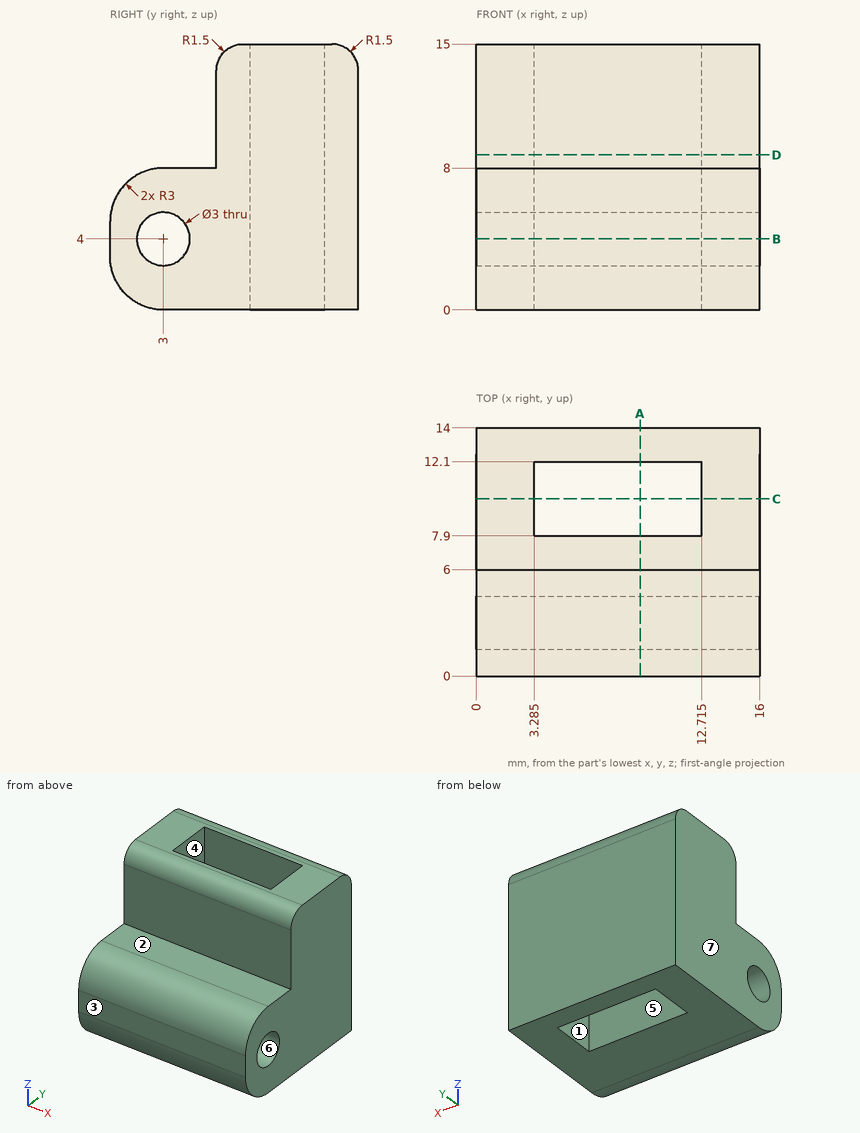
Source: three-view drawing plus pictorial views. Frame: mm from the lowest corner of the part. A direction names the side the tool comes from. Coordinates: 2 decimals unless noted, no trailing zeros. Order: outer loops, then holes, each group sorted by start corner. A loop starts at its lowest first (then second) coordinate and runs counter-clockwise, first axis right, second up. Notation, with made-up numbers: M -37.75,67.25 L 15.25,67.25 A13 ccw 15.25,81.25 Z; hole C 12.25,-34.75 d4. An arc over 180 degrees is marked long. Answer in a Markdown table with one row per item.
(1) Section query A-A, the plane x = 9.25. Output: boundary loops of the cut face in (y, z), plus the area to 3 significant figures.
Numbers:
| item | result |
|---|---|
| outline | M 0,3 A3 ccw 3,0 L 7.9,0 L 7.9,15 L 7.5,15 A1.5 ccw 6,13.5 L 6,8 L 3,8 A3 ccw 0,5 Z; M 12.1,0 L 14,0 L 14,13.5 A1.5 ccw 12.5,15 L 12.1,15 Z; hole C 3,4 d3 |
| area | 93.1 mm^2 |
(2) Section query B-B, the plane z = 4. Output: boundary loops of the cut face in (x, y) (3 decimals), plus the area to 3 significant figures.
Numbers:
| item | result |
|---|---|
| outline | M 0,0 L 16,0 L 16,1.5 L 0,1.5 Z; M 0,4.5 L 16,4.5 L 16,14 L 0,14 Z; hole M 3.285,7.9 L 12.715,7.9 L 12.715,12.1 L 3.285,12.1 Z |
| area | 136 mm^2 |
(3) Access query for the marked faces 1, 2 and 3. Directions: +Z, -Z, +X, -X, +Y, -Y. A direction counts if a zero-diameter tool reaches every point of the face in a straight line with its end or side. Return the directions, or none.
Numbers:
| item | result |
|---|---|
| face 1 | +Z, -Z |
| face 2 | +Z, +X, -X, -Y |
| face 3 | +Z, -Z, +X, -X, -Y |
(4) Section query D-D, the plane z = 8.75. Output: boundary loops of the cut face in (x, y) (3 decimals).
Numbers:
| item | result |
|---|---|
| outline | M 0,6 L 16,6 L 16,14 L 0,14 Z; hole M 3.285,7.9 L 12.715,7.9 L 12.715,12.1 L 3.285,12.1 Z |
(5) Contact query for flat-ended pins moving along their axis: pin 1 Ø1.6 at (x, z) = (6.5, 9.5) entering from -Y; pin 2 Ø0.9 at (x, y) = (8.5, 4.5) entering from +Z; pin 3 Ø1 at (x, z) = (5.5, 8) entering from -Y. Output: stop coordinate, or through.
Numbers:
| item | result |
|---|---|
| pin 1 | stops at y = 6 |
| pin 2 | stops at z = 8 |
| pin 3 | stops at y = 1.34 |
(6) Material intervals for line 1 (X direction, y = 9, z = 10) (3 decimals); line 2 (Z direction, x = 5, y = 3); line 3 (Y direction, x = 8.75, z = 9), sorted ascending. Write a range as [from, to].
Numbers:
| item | result |
|---|---|
| line 1 | x = [0, 3.285], [12.715, 16] |
| line 2 | z = [0, 2.5], [5.5, 8] |
| line 3 | y = [6, 7.9], [12.1, 14] |
(7) Section query C-C, the plane y = 10. Output: boundary loops of the cut face in (x, z) (3 decimals), plus the area to 4 significant figures.
Numbers:
| item | result |
|---|---|
| outline | M 0,0 L 3.285,0 L 3.285,15 L 0,15 Z; M 12.715,0 L 16,0 L 16,15 L 12.715,15 Z |
| area | 98.55 mm^2 |
(8) Draft query along X for the marked faces 4, 5, 6 and 7. Return one class per face: pulls with the +X half, pulls with the -X half, needs draft (parallel to the pull), parting line crosses it, or undercut.
Numbers:
| item | result |
|---|---|
| face 4 | undercut |
| face 5 | undercut |
| face 6 | needs draft |
| face 7 | pulls with the -X half |
